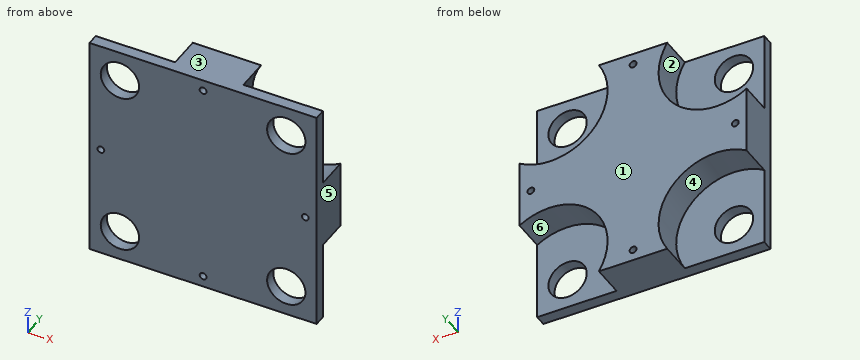
```python
from build123d import *

# Parameters (mm, degrees)
SKETCH1_W               = 100
SKETCH1_H               = 100
SKETCH1_R               = 8.4375
BOSS_EXTRUDE1_DEPTH     = 19.224
SKETCH4_R               = 25.4
CUT_EXTRUDE2_DEPTH      = 14.224
CUT_EXTRUDE1_DEPTH      = 125.005416922
CUT_EXTRUDE1_DEPTH_BACK = 125.005416922
SKETCH3_R               = 1.5


with BuildPart() as part:
    # Sketch1 → Boss-Extrude1 (new body)
    with BuildSketch(Plane(origin=(0, 0, 0), x_dir=(1, 0, 0), z_dir=(0, 1, 0))):
        with Locations((36.625, 36.625)):
            Rectangle(SKETCH1_W, SKETCH1_H)
        with Locations(Location((0, 0, 0), (0, 0, 270))):
            Circle(SKETCH1_R, mode=Mode.SUBTRACT)
        with Locations(Location((0, 73.25, 0), (0, 0, 270))):
            Circle(SKETCH1_R, mode=Mode.SUBTRACT)
        with Locations(Location((73.25, 73.25, 0), (0, 0, 270))):
            Circle(SKETCH1_R, mode=Mode.SUBTRACT)
        with Locations(Location((73.25, 0, 0), (0, 0, 270))):
            Circle(SKETCH1_R, mode=Mode.SUBTRACT)
    extrude(amount=BOSS_EXTRUDE1_DEPTH)

    # Sketch4 → Cut-Extrude2 (cut)
    with BuildSketch(Plane(origin=(0, 19.224, 0), x_dir=(1, 0, 0), z_dir=(0, 1, 0))):
        Circle(SKETCH4_R)
        with Locations((73.25, 0)):
            Circle(SKETCH4_R)
        with Locations((73.25, 73.25)):
            Circle(SKETCH4_R)
        with Locations((0, 73.25)):
            Circle(SKETCH4_R)
    extrude(amount=-CUT_EXTRUDE2_DEPTH, mode=Mode.SUBTRACT)

    # Sketch3 → Cut-Extrude1 (cut, two sides: drawn at the far end of the back side and taken through both)
    with BuildSketch(Plane(origin=(0, 0, 0), x_dir=(1, 0, 0), z_dir=(0, 1, 0)).offset(-CUT_EXTRUDE1_DEPTH_BACK)):
        with Locations(Location((36.625, 81.625, 0), (0, 0, 270))):
            Circle(SKETCH3_R)
        with Locations(Location((81.625, 36.625, 0), (0, 0, 270))):
            Circle(SKETCH3_R)
        with Locations(Location((36.625, -8.375, 0), (0, 0, 270))):
            Circle(SKETCH3_R)
        with Locations(Location((-8.375, 36.625, 0), (0, 0, 270))):
            Circle(SKETCH3_R)
    extrude(amount=CUT_EXTRUDE1_DEPTH + CUT_EXTRUDE1_DEPTH_BACK, mode=Mode.SUBTRACT)


solid = part.part
```
Input: part model. Units: mm. Frame: model coordinates. Face numbers are marked on the shaded views. A direction names the side the tool comes from. Coordinates: 2 decimals unless noted, no trailing zeros. Write each loop counter-clockwise with the first axis right and the second up, starting at its lowest first coordinate (ties: lowest second). Pieces come first, ordered by that corner, then holes. Notation, with made-up numbers: (56.25, 9.5) - (102.25, 9.5) arc R28 cw to (102.25, 41.5) - close; hole circle Ø5 at (54.5, 11). An arc over 180 degrees is marked (long way). Put each result on its own line as item: value. Start each with the question number.
1) Reachability of the marked faces 5 and 6 from +Z, -Z, +X, -X, +Y, -Y: full face, straight path, thin tool, end or side. Return the list, or none.
2) Cut plane C-C (y = 13.75). Return the cut outline in (x, z) (3 decimals).
3) Ray query, L1, parallel to X at y = 2.2, z = -73.25 (1 decimal); L2, parallel to Z at x = 0, y = 3.65 (1 decimal); L3, parallel to Z at x = -4.5, y = 4 (3 decimals). Return the intervals inside material, ascending.
4) Cut plane D-D (x = 60). Return the cut outline in (y, z) (3 decimals), plus the area to 3 significant figures.
5) Contact query for flat-ended pins moving along their axis: pin 1 (1.5 mm diameter, centred on y = 16, z = -14, fed in from -X); pin 2 (19.5 mm diameter, centred on x = 73.25, z = 0, fed in from +Y); pin 3 (3 mm diameter, centred on y = 12, z = -1, fed in from +X). Output: stop coordinate, or through.
6) Mould query, pull axis Z, two halves, no side actions, for the marked faces 1, 2, 3 and 4. Classes: pulls with the +Z half, pulls with the -Z half, needs draft (parallel to the pull), parting line crosses it, or undercut.
7) Cut plane A-A (z = -73.25). State how many separate pieces and enclosed holes the cut face has, plus the area to 3 significant figures.
Resolved:
1. face 5: +Z, -Z, +X, +Y, -Y
1. face 6: +Y
2. outline: (-13.375, -51.657) arc R25.4 cw to (21.593, -86.625) - (51.657, -86.625) arc R25.4 cw to (86.625, -51.657) - (86.625, -21.593) arc R25.4 cw to (51.657, 13.375) - (21.593, 13.375) arc R25.4 cw to (-13.375, -21.593) - close; hole circle Ø3 at (-8.375, -36.625); hole circle Ø3 at (36.625, -81.625); hole circle Ø3 at (36.625, 8.375); hole circle Ø3 at (81.625, -36.625)
3. L1: x = -13.4 to -8.4, 8.4 to 64.8, 81.7 to 86.6
3. L2: z = -86.6 to -81.7, -64.8 to -8.4, 8.4 to 13.4
3. L3: z = -86.625 to -80.387, -66.113 to -7.137, 7.137 to 13.375
4. outline: (0, -86.625) - (5, -86.625) - (5, -51.58) - (19.224, -51.58) - (19.224, -21.67) - (5, -21.67) - (5, 13.375) - (0, 13.375) - close
4. area: 925 mm2
5. pin 1: stops at x = 20.68
5. pin 2: stops at y = 5
5. pin 3: stops at x = 47.97
6. face 1: needs draft
6. face 2: undercut
6. face 3: pulls with the +Z half
6. face 4: undercut
7. separate pieces: 3
7. enclosed holes: 0
7. area: 651 mm2
